Work out the finished part from the listing and answer in its coordinate system (mm). A direction names the side the tool comes from. Give positions to 0.01 mm unless a question says otherwise; leave off trailing zeros. Order: outer loops, then holes, each group sorted by start corner. A loop starts at its lowest first (then second) coordinate and runs counter-clockwise, first axis right, second up. Notation, with made-up numbers: (-14, 0.25) -> (14, 0.25) arc R14 ccw to (14, 18.25) -> close; hole circle Ø9 at (57, -25). An arc over 180 degrees is marked (long way). Use a Markdown table: item, result. Add a question column.
```python
from build123d import *

# Parameters (mm, degrees)
SKETCH1_R             = 2.5
SKETCH1_R_2           = 1
BOSS_EXTRUDE1_DEPTH   = 8
SKETCH1_R_3           = 2.375
SKETCH1_R_4           = 0.875
BOSS_EXTRUDE1_2_DEPTH = 8
SKETCH1_R_5           = 2.25
SKETCH1_R_6           = 0.75
BOSS_EXTRUDE1_3_DEPTH = 8
BOSS_EXTRUDE2_START   = 1.5
SKETCH2_R             = 2.5
SKETCH2_R_2           = 1
BOSS_EXTRUDE2_DEPTH   = 1.5


with BuildPart() as part:
    # Sketch1 → Boss-Extrude1 (new body)
    with BuildSketch(Plane(origin=(0, 0, 0), x_dir=(1, 0, 0), z_dir=(0, 1, 0))):
        with Locations(Location((0, 0, 0), (0, 0, 270))):
            Circle(SKETCH1_R)
        with Locations(Location((0, 0, 0), (0, 0, 270))):
            Circle(SKETCH1_R_2, mode=Mode.SUBTRACT)
    extrude(amount=BOSS_EXTRUDE1_DEPTH)



with BuildPart() as body_2:
    # Sketch1 → Boss-Extrude1 2 (new body)
    with BuildSketch(Plane(origin=(0, 0, 0), x_dir=(1, 0, 0), z_dir=(0, 1, 0))):
        with Locations(Location((6.875, 0, 0), (0, 0, 270))):
            Circle(SKETCH1_R_3)
        with Locations(Location((6.875, 0, 0), (0, 0, 270))):
            Circle(SKETCH1_R_4, mode=Mode.SUBTRACT)
    extrude(amount=BOSS_EXTRUDE1_2_DEPTH)


with BuildPart() as body_3:
    # Sketch1 → Boss-Extrude1 3 (new body)
    with BuildSketch(Plane(origin=(0, 0, 0), x_dir=(1, 0, 0), z_dir=(0, 1, 0))):
        with Locations(Location((13.5, 0, 0), (0, 0, 270))):
            Circle(SKETCH1_R_5)
        with Locations(Location((13.5, 0, 0), (0, 0, 270))):
            Circle(SKETCH1_R_6, mode=Mode.SUBTRACT)
    extrude(amount=BOSS_EXTRUDE1_3_DEPTH)


with BuildPart() as part_1:
    add(part.part)

    add(body_2.part)  # Boss-Extrude2 merges body 2

    add(body_3.part)  # Boss-Extrude2 merges body 3
    # Sketch2 → Boss-Extrude2 (add)
    # profile 1 of 3: a face of its own
    with BuildSketch(Plane.XZ.offset(BOSS_EXTRUDE2_START)):
        Polygon((17.25, 4), (-1.656854249, 4), (-4, 1.656854249), (-4, -4), (17.25, -4), align=None)
        with Locations(Location((0, 0, 0), (0, 0, 270))):
            Circle(SKETCH2_R, mode=Mode.SUBTRACT)
    # profile 2 of 3: a face of its own
    with BuildSketch(Plane.XZ.offset(BOSS_EXTRUDE2_START)):
        with Locations(Location((0, 0, 0), (0, 0, 270))):
            Circle(SKETCH2_R)
        with Locations(Location((0, 0, 0), (0, 0, 90))):
            Circle(SKETCH2_R_2, mode=Mode.SUBTRACT)
    # profile 3 of 3: a face of its own
    with BuildSketch(Plane.XZ.offset(BOSS_EXTRUDE2_START)):
        with Locations(Location((0, 0, 0), (0, 0, 90))):
            Circle(SKETCH2_R_2)
    extrude(amount=-BOSS_EXTRUDE2_DEPTH)


solid = part_1.part
```
1) The part is cut by section C-C, the plane x = 0. Determine the outline of the cut face in (y, z), then the cut area to 3 significant figures.
2) Determine the mould class of faces 3 (the cylindrical face through (-1, 4, 0)), 4 (the cylindrical face through (7.743, 3.944, -0.114)), 5 (the flat face through (17.25, -1, 0)), 6 (the cylindrical face through (-2.44, 3.94, -0.54)) for opening direction Z: released by +Z, released by -Z, zero draft, split by the parting line, or undercut.
3) Flat-ended cylindrical pins translate along their axes: pin 1 (3 mm diameter, centred on x = 9.5, z = -3, fed in from +Y); pin 2 (1.5 mm diameter, centred on x = 0.5, y = 5.5, fed in from +Z). Find the tip coordinate at first contact, or state that the pin passes through.
4) The part is cut by section A-A, the plane z = 0. Determine the outline of the cut face in (x, y).
5) The part is cut by section D-D, the plane z = -1.25. Determine the outline of the cut face in (x, y), then the cut area to 3 significant figures.
6) Straight lines are drawn through the part: line 1 (X direction, y = 2.75, z = 0); line 2 (X direction, y = 6.75, z = -2); line 3 (X direction, y = 4.25, z = 1.5). For each, find the intervals that lie inside material, in ascending order.
7) Which of the six approach directions +Z, -Z, +X, -X, +Y, -Y give full straight-line access (tool end or side, diameter ignored) to faces 1 (the flat face through (8, -1, 4)), 2 (the cylindrical face through (14.244, 3.944, -0.098))?
8) The part is cut by section B-B, the plane y = 7. Determine the outline of the cut face in (x, z) (3 decimals), then the cut area to 3 significant figures.
A:
| question | item | result |
|---|---|---|
| 1 | outline | (-1.5, -4) -> (0, -4) -> (0, -2.5) -> (8, -2.5) -> (8, -1) -> (0, -1) -> (0, 1) -> (8, 1) -> (8, 2.5) -> (0, 2.5) -> (0, 4) -> (-1.5, 4) -> close |
| 1 | area | 36.0 mm^2 |
| 2 | face 3 | undercut |
| 2 | face 4 | undercut |
| 2 | face 5 | zero draft |
| 2 | face 6 | split by the parting line |
| 3 | pin 1 | y = 0 |
| 3 | pin 2 | z = 2.5 |
| 4 | outline | (-4, -1.5) -> (17.25, -1.5) -> (17.25, 0) -> (15.75, 0) -> (15.75, 8) -> (14.25, 8) -> (14.25, 0) -> (12.75, 0) -> (12.75, 8) -> (11.25, 8) -> (11.25, 0) -> (9.25, 0) -> (9.25, 8) -> (7.75, 8) -> (7.75, 0) -> (6, 0) -> (6, 8) -> (4.5, 8) -> (4.5, 0) -> (2.5, 0) -> (2.5, 8) -> (1, 8) -> (1, 0) -> (-1, 0) -> (-1, 8) -> (-2.5, 8) -> (-2.5, 0) -> (-4, 0) -> close |
| 5 | outline | (-4, -1.5) -> (17.25, -1.5) -> (17.25, 0) -> (15.37, 0) -> (15.37, 8) -> (11.63, 8) -> (11.63, 0) -> (8.89, 0) -> (8.89, 8) -> (4.86, 8) -> (4.86, 0) -> (2.17, 0) -> (2.17, 8) -> (-2.17, 8) -> (-2.17, 0) -> (-4, 0) -> close |
| 5 | area | 129 mm^2 |
| 6 | line 1 | -2.5 to -1, 1 to 2.5, 4.5 to 6, 7.75 to 9.25, 11.25 to 12.75, 14.25 to 15.75 |
| 6 | line 2 | -1.5 to 1.5, 5.59 to 8.16, 12.47 to 14.53 |
| 6 | line 3 | -2 to 2, 5.03 to 8.72, 11.82 to 15.18 |
| 7 | face 1 | +Z, +X, -X, +Y, -Y |
| 7 | face 2 | +Y |
| 8 | outline | circle Ø5 at (0, 0); circle Ø4.75 at (6.875, 0); circle Ø4.5 at (13.5, 0); hole circle Ø2 at (0, 0); hole circle Ø1.75 at (6.875, 0); hole circle Ø1.5 at (13.5, 0) |
| 8 | area | 45.9 mm^2 |
